from build123d import *

# Parameters (mm, degrees)
BOSS_EXTRUDE1_DEPTH = 500
SKETCH2_R           = 12.5
CUT_EXTRUDE1_DEPTH  = 485.648
SKETCH3_W           = 500
SKETCH3_H           = 6.4
BOSS_EXTRUDE3_DEPTH = 20
SKETCH4_W           = 500
SKETCH4_H           = 6.4
BOSS_EXTRUDE4_DEPTH = 20
BOSS_EXTRUDE5_DEPTH = 6.4
SKETCH6_W           = 288.065528703
SKETCH6_H           = 25.425
BOSS_EXTRUDE6_DEPTH = 6.4


with BuildPart() as part:
    # Sketch1 → Boss-Extrude1 (new body)
    with BuildSketch(Plane.XY):
        Polygon((-69.85, 19.05), (-69.85, -19.049737181), (69.85, -19.049737181), (205.465528703, -19.049737181), (205.465528703, 19.05), (211.865528703, 19.05), (211.865528703, -25.4), (76.2, -25.4), (-76.2, -25.4), (-76.2, 19.05), align=None)
    extrude(amount=BOSS_EXTRUDE1_DEPTH)

    # Sketch2 → Cut-Extrude1 (cut)
    with BuildSketch(Plane(origin=(211.865528703, 0, 0), x_dir=(0, 0, -1), z_dir=(1, 0, 0))):
        with Locations(Location((-400, -3.2, 0), (0, 0, 180))):
            Circle(SKETCH2_R)
        with Locations(Location((-100, -3.2, 0), (0, 0, 180))):
            Circle(SKETCH2_R)
    extrude(amount=-CUT_EXTRUDE1_DEPTH, mode=Mode.SUBTRACT)

    # Sketch3 → Boss-Extrude3 (add)
    with BuildSketch(Plane(origin=(211.865528703, 0, 0), x_dir=(0, 0, -1), z_dir=(1, 0, 0))):
        with Locations((-250, 22.25)):
            Rectangle(SKETCH3_W, SKETCH3_H)
    extrude(amount=-BOSS_EXTRUDE3_DEPTH)

    # Sketch4 → Boss-Extrude4 (add)
    with BuildSketch(Plane.ZY.offset(76.2)):
        with Locations((250, 22.25)):
            Rectangle(SKETCH4_W, SKETCH4_H)
    extrude(amount=-BOSS_EXTRUDE4_DEPTH)

    # Sketch5 → Boss-Extrude5 (add)
    with BuildSketch(Plane(origin=(0, 0, 0), x_dir=(-1, 0, 0), z_dir=(0, 0, -1))):
        Polygon((-211.865528703, -25.4), (76.2, -25.4), (76.2, -19.058688743), (76.2, 0.025), (69.85, 0.00013141), (-205.465528703, 0.00013141), (-211.865528703, 0.025), (-211.865528703, -19.058688743), align=None)
    extrude(amount=BOSS_EXTRUDE5_DEPTH)

    # Sketch6 → Boss-Extrude6 (add)
    with BuildSketch(Plane.XY.offset(500)):
        with Locations((67.832764352, -12.6875)):
            Rectangle(SKETCH6_W, SKETCH6_H)
    extrude(amount=BOSS_EXTRUDE6_DEPTH)


solid = part.part
The listing builds one solid part. Answer for the finished solid, in the listing's coordinates (mm). A direction names the side the tool comes from. Give positions to 0.01 mm unless a question says otherwise; leave off trailing zeros. Loops run counter-clockwise (first coordinate to the right, second up) from the corner with the lowest first, then second, coordinate; pieces in that order, holes last.
Item 1: Determine the mould class of faces 1 (the flat face through (-66, 25.45, 247)), 2 (the cylindrical face through (208.71, -6.955, 411.923)), 3 (the flat face through (-71, 15, 500)) for opening direction Y: +Y half, -Y half, draft (parallel to the pull), parting line (faces both ways), or undercut.
Derived:
face 1: +Y half
face 2: undercut
face 3: draft
Item 2: A cutting plane is placed at C-C (z = 266.5). Give the vertices of the cut face in (x, y).
Derived:
outline: (-76.2, -25.4) - (211.87, -25.4) - (211.87, 25.45) - (191.87, 25.45) - (191.87, 19.05) - (205.47, 19.05) - (205.47, -19.05) - (-69.85, -19.05) - (-69.85, 19.05) - (-56.2, 19.05) - (-56.2, 25.45) - (-76.2, 25.45) - close
Item 3: A cutting plane is placed at B-B (x = 167). Give the vertices of the cut face in (y, z) (3 decimals).
Derived:
outline: (-25.4, -6.4) - (0, -6.4) - (0, 0) - (-19.05, 0) - (-19.05, 500) - (0.025, 500) - (0.025, 506.4) - (-25.4, 506.4) - close
Item 4: A cutting plane is placed at A-A (z = 400). Give the vertices of the cut face in (x, y), then the cut area to 3 significant figures.
Derived:
outline: (-76.2, -25.4) - (211.87, -25.4) - (211.87, -15.7) - (205.47, -15.7) - (205.47, -19.05) - (-69.85, -19.05) - (-69.85, -15.7) - (-76.2, -15.7) - close; (-76.2, 9.3) - (-69.85, 9.3) - (-69.85, 19.05) - (-56.2, 19.05) - (-56.2, 25.45) - (-76.2, 25.45) - close; (191.87, 19.05) - (205.47, 19.05) - (205.47, 9.3) - (211.87, 9.3) - (211.87, 25.45) - (191.87, 25.45) - close
area: 2,250 mm2
Item 5: Find the intervals of material crossed by line 1 along Y through (x, z) = (209.5, 100); line 2 along X through (y, z) = (-3, 254.5); line 3 along Z through (x, y) = (81, -13.5), in increasing order.
Derived:
line 1: y = -25.4 to -15.7, 9.3 to 25.45
line 2: x = -76.2 to -69.85, 205.47 to 211.87
line 3: z = -6.4 to 0, 500 to 506.4
Item 6: A tool of negligible diameter and unlimited length cuts with its end or side. For faces 4 (the flat face through (-69.85, 0, 246)), 5 (the flat face through (206, 15, 500)), 6 (the flat face through (66, -25.4, 246)), 7 (the flat face through (199, 19.05, 253)), 8 (the flat face through (-71, 15, 0)), from which of +Z, -Z, +X, -X, +Y, -Y can it reach the whole face along a straight path? Write none if from no direction.
Derived:
face 4: none
face 5: +Z, +X, -X, +Y
face 6: +Z, -Z, +X, -X, -Y
face 7: +Z, -Z
face 8: -Z, +X, -X, +Y
Item 7: Each of these flat-tipped pins is pushed along its axis until it touches: pin 1 Ø3 at (x, z) = (42.5, 502) entering from +Y (3 decimals); pin 2 Ø22.5 at (y, z) = (-3.2, 400) entering from +X; pin 3 Ø10 at (x, y) = (-70, 15) entering from +Z; pin 4 Ø12 at (x, z) = (138.5, 442.5) entering from +Y. Where does it stop, or does it pass through?
Derived:
pin 1: stops at y = 0.025
pin 2: passes through
pin 3: stops at z = 500
pin 4: stops at y = -19.05
